```python
from build123d import *

# Parameters (mm, degrees)
F0_W            = 43.0059846
F0_H            = 43.0059846
F0_R            = 1.5
F0_R_2          = 11.2530001
F1_DEPTH        = 1.58115
F2_SIZE         = 6.0030106
F4_DEPTH        = 1.58115
F4_COPIES_COUNT = 4


# Not quite as in the source:
# - a pattern or mirror of a feature is missing from the dataset's text; its kind, count and spacing are read off the source's solid


with BuildPart() as f1:
    # F0 (on Top) → F1 (new body)
    with BuildSketch(Plane.XY):
        with Locations((21.5029923, 21.5029923)):
            Rectangle(F0_W, F0_H)
        with Locations((6.0029979, 6.0029979)):
            Circle(F0_R, mode=Mode.SUBTRACT)
        with Locations((21.5029923, 21.5029923)):
            Circle(F0_R_2, mode=Mode.SUBTRACT)
        with Locations((37.0029867, 6.0029979)):
            Circle(F0_R, mode=Mode.SUBTRACT)
        with Locations((6.0029979, 37.0029867)):
            Circle(F0_R, mode=Mode.SUBTRACT)
        with Locations((37.0029867, 37.0029867)):
            Circle(F0_R, mode=Mode.SUBTRACT)
    extrude(amount=F1_DEPTH)

    # F2
    f2_edges = [f1.edges().sort_by_distance(p)[0] for p in [
        (0, 0, 0.790575),
        (0, 43.005985, 0.790575),
        (43.005985, 0, 0.790575),
        (43.005985, 43.005985, 0.790575),
    ]]
    chamfer(f2_edges, length=F2_SIZE)

    # F3 (on face) → F4 (cut, through all)
    with BuildSketch(Plane.XY.offset(1.58115)):
        with BuildLine():
            ThreePointArc((7.2356236023, 32.4027649523), (5.1176370603, 32.3235056996), (3.175, 33.171037571))
            Line((3.175, 33.171037571), (3.175, 9.834947029))
            ThreePointArc((3.175, 9.834947029), (5.1176370603, 10.6824789004), (7.2356236023, 10.6032196477))
            Line((7.2356236023, 10.6032196477), (9.7569670059, 13.1245630513))
            ThreePointArc((9.7569670059, 13.1245630513), (7.0749922, 21.5029923), (9.7569670059, 29.8814215487))
            Line((9.7569670059, 29.8814215487), (7.2356236023, 32.4027649523))
        make_face()
    f4 = extrude(amount=-F4_DEPTH, mode=Mode.SUBTRACT)

    # F4_copies: F4 ×4 about axis
    f4_copies_axis = Axis((21.502992, 21.502992, 0), (0, 0, 1))
    for i in range(1, F4_COPIES_COUNT):
        add(f4.rotate(f4_copies_axis, i * 360 / F4_COPIES_COUNT), mode=Mode.SUBTRACT)


solid = f1.part
```
Input: part model. Units: mm. Frame: model coordinates. A direction names the side the tool comes from. Give positions to 0.01 mm unless a question says otherwise; leave off trailing zeros. Order: outer loops, then holes, each group sorted by start corner. A loop starts at its lowest first (then second) coordinate and runs counter-clockwise, first axis right, second up. Notation, with made-up numbers: (25.25, 86.5) - (45.25, 86.5) arc R13 cw to (45.25, 90.5) - close; hole circle Ø3 at (5, 50.25). An arc over 180 degrees is marked (long way). One line per item, written item: value.
1. Pin query (flat end, axial travel): pin 1 Ø1.5 at (x, y) = (8.5, 34.5) entering from -Z. Return the tip coordinate at first contact, or that it passes through.
Determined:
pin 1: z = 0
2. Cut plane A-A, the plane x = 27.5. Output: boundary loops of the cut face in (y, z) (3 decimals), and give its area (3 significant figures).
Determined:
outline: (0, 0) - (3.175, 0) - (3.175, 1.581) - (0, 1.581) - close; (8.38, 0) - (11.981, 0) - (11.981, 1.581) - (8.38, 1.581) - close; (31.025, 0) - (34.626, 0) - (34.626, 1.581) - (31.025, 1.581) - close; (39.831, 0) - (43.006, 0) - (43.006, 1.581) - (39.831, 1.581) - close
area: 21.4 mm2
3. Reachability of faces 1 (the face through (21, 0, 1)), 2 (the face through (39.831, 21, 1)) from +Z, -Z, +X, -X, +Y, -Y: full face, straight path, thin tool, end or side. Return the list, or none.
Determined:
face 1: +Z, -Z, +X, -X, -Y
face 2: +Z, -Z
4. Line query: probe 1 along X at (y, z) = (21, 0.85) (3 decimals); probe 2 along X at (y, z) = (6, 0.25); probe 3 along Y at (x, z) = (19, 0.4) (3 decimals). Output: solid intervals per line, ascending.
Determined:
probe 1: 0 to 3.175, 7.084 to 10.261, 32.745 to 35.922, 39.831 to 43.006
probe 2: 0 to 4.5, 7.5 to 10.77, 32.24 to 35.5, 38.5 to 43
probe 3: 0 to 3.175, 7.294 to 10.532, 32.474 to 35.712, 39.831 to 43.006
5. Cut plane D-D, the plane x = 35. Output: boundary loops of the cut face in (y, z).
Determined:
outline: (0, 0) - (11.37, 0) - (11.37, 1.58) - (0, 1.58) - close; (16.4, 0) - (26.6, 0) - (26.6, 1.58) - (16.4, 1.58) - close; (31.63, 0) - (43.01, 0) - (43.01, 1.58) - (31.63, 1.58) - close
6. Draft query along X for faces 3 (the face through (0, 21, 1)), 4 (the face through (34.53, 31.16, 0.8)), 5 (the face through (5.088, 10.677, 0.802)), 6 (the face through (43.006, 21, 1)). Return one class per face: released by +X, released by -X, zero draft, split by the parting line, or undercut.
Determined:
face 3: released by -X
face 4: undercut
face 5: undercut
face 6: released by +X
7. Cut plane B-B, the plane y = 17. Output: boundary loops of the cut face in (x, z) (3 decimals), and give its area (3 significant figures).
Determined:
outline: (0, 0) - (3.175, 0) - (3.175, 1.581) - (0, 1.581) - close; (7.796, 0) - (11.19, 0) - (11.19, 1.581) - (7.796, 1.581) - close; (31.816, 0) - (35.21, 0) - (35.21, 1.581) - (31.816, 1.581) - close; (39.831, 0) - (43.006, 0) - (43.006, 1.581) - (39.831, 1.581) - close
area: 20.8 mm2
8. Cut plane C-C, the plane y = 39. Output: boundary loops of the cut face in (x, z).
Determined:
outline: (2, 0) - (10.33, 0) - (10.33, 1.58) - (2, 1.58) - close; (32.68, 0) - (41.01, 0) - (41.01, 1.58) - (32.68, 1.58) - close
